Could you check a few things on this model? Use its own coordinates, in mm. A direction names the side the tool comes from. Round coordinates to 2 decimals unless told otherwise and drop trailing zeros. Write each loop counter-clockwise with the first axis right and the second up, starting at its lowest first coordinate (ties: lowest second). Pieces come first, ordered by that corner, then holes. Notation, with made-up numbers: (11, -5) -> (24, -5) arc R28 ccw to (24, 15) -> close; hole circle Ø5 at (-12.75, -31). An arc over 180 degrees is marked (long way). Answer in a Markdown table with one row per item.
from build123d import *

# Parameters (mm, degrees)
SKETCH1_R           = 2.5
SKETCH1_R_2         = 2.25
SKETCH1_R_3         = 3
SKETCH1_R_4         = 2.2
BOSS_EXTRUDE1_DEPTH = 5


with BuildPart() as part:
    # Sketch1 → Boss-Extrude1 (new body)
    with BuildSketch(Plane(origin=(0, 0, 0), x_dir=(1, 0, 0), z_dir=(0, 1, 0))):
        Polygon((-91.72214446, -4.653561253), (-91.72214446, 90.346388656), (-23.72214446, 262.395827557), (-13.72214446, 262.395827557), (-13.72214446, 211.395827557), (-41.469832452, 121.346438747), (42.025543532, 121.346438747), (14.27785554, 211.395827557), (14.27785554, 262.395827557), (24.27785554, 262.395827557), (92.27785554, 90.346388656), (92.27785554, -4.653561253), (92.27785554, -10.433561253), (92.27785554, -14.668275992), (72.27785554, -14.668275992), (72.27785554, -10.433561253), (72.27785554, -4.653561253), (72.27785554, 11.346431169), (81.27785554, 11.346431169), (81.27785554, 64.346431169), (17.277798113, 64.346431169), (17.277798113, -4.653561253), (17.277798113, -10.433561253), (17.277798113, -14.668275992), (-91.456714597, -14.668275992), (-91.72214446, -14.668275992), (-91.72214446, -10.433561253), align=None)
        with Locations(Location((77.010414368, 0.346438747, 0), (0, 0, 270))):
            Circle(SKETCH1_R, mode=Mode.SUBTRACT)
        with Locations(Location((77.010414368, 80.346438747, 0), (0, 0, 270))):
            Circle(SKETCH1_R, mode=Mode.SUBTRACT)
        with Locations(Location((21.010414368, 80.346438747, 0), (0, 0, 270))):
            Circle(SKETCH1_R, mode=Mode.SUBTRACT)
        with Locations(Location((-18.72214446, 257.395827557, 0), (0, 0, 270))):
            Circle(SKETCH1_R_2, mode=Mode.SUBTRACT)
        with Locations(Location((-18.72214446, 216.395827557, 0), (0, 0, 270))):
            Circle(SKETCH1_R_2, mode=Mode.SUBTRACT)
        with Locations(Location((19.27785554, 257.395827557, 0), (0, 0, 270))):
            Circle(SKETCH1_R_2, mode=Mode.SUBTRACT)
        with Locations(Location((19.27785554, 216.395827557, 0), (0, 0, 270))):
            Circle(SKETCH1_R_2, mode=Mode.SUBTRACT)
        with Locations(Location((-37.72214446, 191.551940951, 0), (0, 0, 270))):
            Circle(SKETCH1_R_3, mode=Mode.SUBTRACT)
        with Locations(Location((38.27785554, 191.551940951, 0), (0, 0, 270))):
            Circle(SKETCH1_R_3, mode=Mode.SUBTRACT)
        with Locations(Location((-72.656714597, -5.450648645, 0), (0, 0, 270))):
            Circle(SKETCH1_R_4, mode=Mode.SUBTRACT)
        with Locations(Location((-72.656714597, 30.549351355, 0), (0, 0, 270))):
            Circle(SKETCH1_R_4, mode=Mode.SUBTRACT)
    extrude(amount=BOSS_EXTRUDE1_DEPTH)


solid = part.part
1) Imagine slicing it at A-A, the plane z = -56.5. Please give me the cut outline in (x, y).
Findings:
| item | result |
|---|---|
| outline | (-91.72, 0) -> (17.28, 0) -> (17.28, 5) -> (-91.72, 5) -> close; (81.28, 0) -> (92.28, 0) -> (92.28, 5) -> (81.28, 5) -> close |
2) Imagine slicing it at C-C, the plane z = -246. Please give me the cut outline in (x, y).
Findings:
| item | result |
|---|---|
| outline | (-30.2, 0) -> (-13.72, 0) -> (-13.72, 5) -> (-30.2, 5) -> close; (14.28, 0) -> (30.76, 0) -> (30.76, 5) -> (14.28, 5) -> close |
3) For faces 1 (the face through (-91.722, 2, -39)), 2 (the face through (19, 2, -262.396)), 3 (the face through (17.278, 2, -24)), 4 (the face through (28.346, 2.465, -165.741)), 5 (the face through (-13.722, 2, -237)), which set-ups out of +Z, -Z, +X, -X, +Y, -Y let a thin tool reach every point of the face, with its end or its side?
Findings:
| item | result |
|---|---|
| face 1 | +Z, -Z, -X, +Y, -Y |
| face 2 | -Z, +X, -X, +Y, -Y |
| face 3 | +Z, +Y, -Y |
| face 4 | +Y, -Y |
| face 5 | -Z, +Y, -Y |
4) Imagine slicing it at B-B, the plane y = 3.7. Count the separate pieces of the cut face and the enclosed holes in it, plus the area to 3 significant figures.
Findings:
| item | result |
|---|---|
| separate pieces | 1 |
| enclosed holes | 11 |
| area | 27,800 mm^2 |
5) Please list where these lines run through material, in increasing order: line 1 (X direction, y = 0.5, z = -11.5); line 2 (X direction, y = 3.35, z = 0.5); line 3 (Z direction, x = -1.5, y = 2.4).
Findings:
| item | result |
|---|---|
| line 1 | x = -91.72 to 17.28, 81.28 to 92.28 |
| line 2 | x = -91.72 to 17.28, 72.28 to 74.66, 79.36 to 92.28 |
| line 3 | z = -121.35 to 14.67 |
6) For pin 1 (10 mm diameter, centred on x = 68, z = -69, fed in from -Y); pin 2 (3 mm diameter, centred on x = 65, y = 1.5, fed in from +Z), each with a flat end and sliding along its axis, tell me the tip position at first contact or that it passes through.
Findings:
| item | result |
|---|---|
| pin 1 | stops at y = 0 |
| pin 2 | stops at z = -64.35 |
7) Imagine slicing it at D-D, the plane x = 8.5. Please give me the cut outline in (y, z), plus the area to 3 significant figures.
Findings:
| item | result |
|---|---|
| outline | (0, -121.35) -> (5, -121.35) -> (5, 14.67) -> (0, 14.67) -> close |
| area | 680 mm^2 |
